from build123d import *

# Parameters (mm, degrees)
EXTRUDE_1_DEPTH     = 10
SKETCH_2_R          = 3.65
CUT_EXTRUDE_1_DEPTH = 4
CUT_EXTRUDE_2_REACH = 5
SKETCH_3_R          = 2.25
SKETCH_4_R          = 3.4
FILLET_1_R          = 5
FILLET_2_R          = 10


with BuildPart() as part:
    # 草圖1 → 填料-伸長1 (new body, symmetric)
    with BuildSketch(Plane.XY):
        Polygon((20, 0), (20, 25), (0, 25), (0, 7), (-20, 7), (-20, 0), align=None)
    extrude(amount=EXTRUDE_1_DEPTH, both=True)

    # 草圖2 → 除料-伸長1 (cut)
    with BuildSketch(Plane(origin=(0, 7, 0), x_dir=(1, 0, 0), z_dir=(0, 1, 0))):
        with Locations((-10, 0)):
            Circle(SKETCH_2_R)
    extrude(amount=-CUT_EXTRUDE_1_DEPTH, mode=Mode.SUBTRACT)

    # 草圖3 → 除料-伸長2 (cut, up to next)
    with BuildSketch(Plane(origin=(0, 3, 0), x_dir=(1, 0, 0), z_dir=(0, 1, 0)), mode=Mode.PRIVATE) as cut_extrude_2_sk1:
        with Locations((-10, 0)):
            Circle(SKETCH_3_R)
    cut_extrude_2_tool1 = extrude(cut_extrude_2_sk1.sketch, amount=-CUT_EXTRUDE_2_REACH, mode=Mode.PRIVATE) & part.part
    add(cut_extrude_2_tool1.solids().sort_by_distance((-10, 3, 0))[0], mode=Mode.SUBTRACT)

    # 除料-掃出1: sweep along a path in 草圖5
    with BuildLine(Plane(origin=(10, 0, 10), x_dir=(0, 0, -1), z_dir=(1, 0, 0))) as sweep_1_path:
        Line((10, 0), (10, 12))
        ThreePointArc((10, 12), (12.343145751, 17.656854249), (18, 20))
        Line((18, 20), (20, 20))
    # 草圖4 → 除料-掃出1 (sweep, cut)
    with BuildSketch(Plane.XZ):
        with Locations((10, 0)):
            Circle(SKETCH_4_R)
    sweep(path=sweep_1_path.line, mode=Mode.SUBTRACT)

    # 圓角1
    fillet_1_edges = [part.edges().sort_by_distance(p)[0] for p in [
        (0, 7, 0),
    ]]
    fillet(fillet_1_edges, radius=FILLET_1_R)

    # 圓角2
    fillet_2_edges = [part.edges().sort_by_distance(p)[0] for p in [
        (0, 25, 0),
    ]]
    fillet(fillet_2_edges, radius=FILLET_2_R)


solid = part.part
Source: CAD feature listing. Evaluate the final solid. Frame: model axes, mm. A direction names the side the tool comes from. Coordinates: 2 decimals unless noted, no trailing zeros. Write each loop counter-clockwise with the first axis right and the second up, starting at its lowest first coordinate (ties: lowest second). Pieces come first, ordered by that corner, then holes. Notation, with made-up numbers: M 63,24 L 72,24 A3 cw 72,29 Z; hole C -24,20.5 d8. An arc over 180 degrees is marked long. Use a Markdown table: item, result.
1) Section C-C, the plane z = 5.75. Output: boundary loops of the cut face in (x, y).
Conclusion:
| item | result |
|---|---|
| outline | M -20,0 L 20,0 L 20,25 L 10,25 A10 ccw 0,15 L 0,12 A5 cw -5,7 L -20,7 Z |
2) First-contact query: pin 1 Ø2 at (x, z) = (-11.5, 0.5) entering from +Y; pin 2 Ø12 at (x, z) = (-12, -0.5) entering from +Y; pin 3 Ø1.5 at (x, z) = (5.5, -3) entering from +Y. Flat tips, straight axial feed; report the tip coordinate or a pass-through.
Conclusion:
| item | result |
|---|---|
| pin 1 | stops at y = 3 |
| pin 2 | stops at y = 7 |
| pin 3 | stops at y = 24.27 |
3) Reachability of faces 1 (the cylindrical face through (-13.646, 5.028, -0.16)), 2 (the flat face through (-14, 7, 0)), 3 (the cylindrical face through (13.14, 6.08, 1.3)) from +Z, -Z, +X, -X, +Y, -Y: full face, straight path, thin tool, end or side. Return the list, or none.
Conclusion:
| item | result |
|---|---|
| face 1 | +Y |
| face 2 | +Z, -Z, -X, +Y |
| face 3 | -Y |
4) Section D-D, the plane x = -1. Output: boundary loops of the cut face in (y, z), then the cut area to 3 significant figures.
Conclusion:
| item | result |
|---|---|
| outline | M 0,-10 L 9,-10 L 9,10 L 0,10 Z |
| area | 180 mm^2 |
5) Mould query, pull axis Z, two halves, no side actions, for faces 4 (the flat face through (-12, 3, 2)), 5 (the cylindrical face through (11.6, 23, -9)), 6 (the flat face through (4, 10, -10)). Classes: pulls with the +Z half, pulls with the -Z half, needs draft (parallel to the pull), parting line crosses it, or undercut.
Conclusion:
| item | result |
|---|---|
| face 4 | undercut |
| face 5 | needs draft |
| face 6 | pulls with the -Z half |
6) Section B-B, the plane y = 9. Output: boundary loops of the cut face in (x, z).
Conclusion:
| item | result |
|---|---|
| outline | M -1,-10 L 20,-10 L 20,10 L -1,10 Z; hole C 10,0 d6.8 |
7) Section A-A, the plane y = 3.75. Output: boundary loops of the cut face in (x, z).
Conclusion:
| item | result |
|---|---|
| outline | M -20,-10 L 20,-10 L 20,10 L -20,10 Z; hole C -10,0 d7.3; hole C 10,0 d6.8 |
8) Ray query, L1, parallel to X at y = 2.2, z = 0; L2, parallel to Z at x = 10, y = 9.25; L3, parallel to Y at x = 10, z = -9.15. Return the intervals inside material, ascending.
Conclusion:
| item | result |
|---|---|
| L1 | x = -20 to -12.25, -7.75 to 6.6, 13.4 to 20 |
| L2 | z = -10 to -3.4, 3.4 to 10 |
| L3 | y = 0 to 16.6, 23.4 to 25 |
